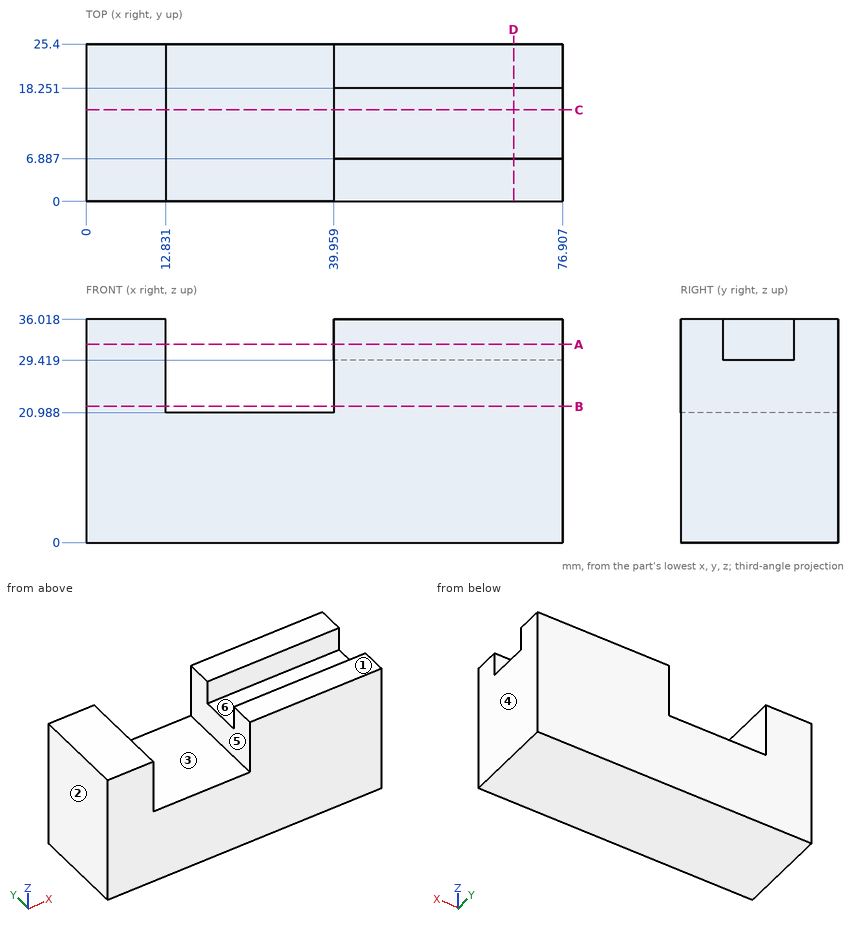
Design review of the part shown in the three views and the two pictorial views. Dimensions are in mm from the part's minimum x, y and z. A direction names the side the tool comes from. Give positions to 0.01 mm unless a question says otherwise; leave off trailing zeros. Loops run counter-clockwise (first coordinate to the right, second up) from the corner with the lowest first, then second, coordinate; pieces in that order, holes last. Notation, with made-up numbers: M 46,67 L 92,67 A6 ccw 92,76 Z; hole C -5.5,67.25 d10. An arc over 180 degrees is marked long. Write item = value, one per line.
Q1. We need section B-B (z = 22). Give the boundary of the cut face in (x, y).
Output values:
outline = M 0,0 L 12.83,0 L 12.83,25.4 L 0,25.4 Z; M 39.96,0 L 76.91,0 L 76.91,25.4 L 39.96,25.4 Z
Q2. Draft analysis for pull direction X (two halves, no side actions). For the marked faces 1, 2 and 3, state which applies: +X half, -X half, draft (parallel to the pull), parting line (faces both ways), or undercut.
Output values:
face_1 = draft
face_2 = -X half
face_3 = undercut
Q3. We need section A-A (z = 32). Give the boundary of the cut face in (x, y).
Output values:
outline = M 0,0 L 12.83,0 L 12.83,25.4 L 0,25.4 Z; M 39.96,0 L 76.91,0 L 76.91,6.89 L 39.96,6.89 Z; M 39.96,18.25 L 76.91,18.25 L 76.91,25.4 L 39.96,25.4 Z
Q4. We need section D-D (x = 69). Give the boundary of the cut face in (y, z), plus the area to 3 significant figures.
Output values:
outline = M 0,0 L 25.4,0 L 25.4,36.02 L 18.25,36.02 L 18.25,29.42 L 6.89,29.42 L 6.89,36.02 L 0,36.02 Z
area = 840 mm^2
Q5. For the marked faces 4, 5 and 6, list the 3-axis set-ups (+Z, -Z, +X, -X, +Y, -Y) from which the entire face can be reached by the end or side of a thin tool; tool diameter is ignored.
Output values:
face_4 = +Z, -Z, +X, +Y, -Y
face_5 = +Z, +Y, -Y
face_6 = +Z, +X
Q6. Insertion check: pin 1 (1 mm diameter, centred on x = 59, y = 10, fed in from +Z). The pin has a flat end and moves straight along its axis. Give the tip position at first contact, or say it passes through.
Output values:
pin_1 = 29.42
Q7. We need section C-C (y = 14.75). Give the boundary of the cut face in (x, z).
Output values:
outline = M 0,0 L 76.91,0 L 76.91,29.42 L 39.96,29.42 L 39.96,20.99 L 12.83,20.99 L 12.83,36.02 L 0,36.02 Z
Q8. To check wall thickness, follow line 1 (X direction, y = 20.75, z = 28); line 2 (Y direction, x = 51.5, z = 31); line 3 (Z direction, x = 53, y = 16.25). State the ranges of each line that lie inside material, in increasing order. Write a range as [from, to].
Output values:
line_1 = [0, 12.83], [39.96, 76.91]
line_2 = [0, 6.89], [18.25, 25.4]
line_3 = [0, 29.42]
